Here's how the part is built. I have some questions about the finished solid (model axes, mm). Face numbers are marked on the shaded views. A direction names the side the tool comes from. Coordinates: 2 decimals unless noted, no trailing zeros. Write each loop counter-clockwise with the first axis right and the second up, starting at its lowest first coordinate (ties: lowest second). Pieces come first, ordered by that corner, then holes. Notation, with made-up numbers: (-4.5, -1) - (41.5, -1) arc R28 cw to (41.5, 32) - close; hole circle Ø8 at (-21.75, 9.25). An arc over 180 degrees is marked (long way). Answer in a Markdown table with one row per item. Add a question column.
Item 1: If I drill on probe 1 along X at (y, z) = (-10, -28); probe 2 along Z at (x, y) = (37, 12); probe 3 along Y at (x, z) = (90, -23), over which ranges is the centre line in solid material (lowest first)? Write a range as from..to.
Item 2: Imagine slicing it at A-A (y = 0). Please give me the cut outline in (x, z), plus the area to 3 significant figures.
Item 3: Imagine slicing it at C-C (x = 125.5). Please give me the cut outline in (y, z), plus the area to 3 significant figures.
Item 4: Imagine slicing it at D-D (y = 22). Please give me the cut outline in (x, z).
Item 5: Which directions (+Z, -Z, +X, -X, +Y, -Y) give clear straight access to the entire face, cutting with the end or side of a thin tool? Please do the marked faces 1 and 2.
Item 6: I'm going to push flat-ended pins straight in: pin 1 (12 mm diameter, centred on y = -4, z = -31, fed in from +X); pin 2 (6 mm diameter, centred on x = 84.5, z = 14, fed in from +Y); pin 3 (5 mm diameter, centred on x = 96.5, z = -17, fed in from -Y). Where does each tip first touch, or does it pass through?
from build123d import *

# Parameters (mm, degrees)
F0_R     = 40.5
F1_DEPTH = 100
F2_W     = 90
F2_H     = 90
F3_DEPTH = 100.001
F4_R     = 10
F5_DEPTH = 40


with BuildPart() as f1:
    # F0 (on Right) → F1 (new body)
    with BuildSketch(Plane.YZ):
        Circle(F0_R)
    extrude(amount=F1_DEPTH)

    # F2 (on face) → F3 (cut, through all)
    with BuildSketch(Plane.YZ.offset(100)):
        Rectangle(F2_W, F2_H)
        with BuildLine():
            Line((40, -6.3442887702), (40, -40))
            Line((40, -40), (6.3442887702, -40))
            ThreePointArc((6.3442887702, -40), (0, -40.5), (-6.3442887702, -40))
            Line((-6.3442887702, -40), (-40, -40))
            Line((-40, -40), (-40, -6.3442887702))
            ThreePointArc((-40, -6.3442887702), (-40.5, 0), (-40, 6.3442887702))
            Line((-40, 6.3442887702), (-40, 40))
            Line((-40, 40), (-6.3442887702, 40))
            ThreePointArc((-6.3442887702, 40), (0, 40.5), (6.3442887702, 40))
            Line((6.3442887702, 40), (40, 40))
            Line((40, 40), (40, 6.3442887702))
            ThreePointArc((40, 6.3442887702), (40.3748065011, 3.1819805153), (40.5, 0))
            ThreePointArc((40.5, 0), (40.3748065011, -3.1819805153), (40, -6.3442887702))
        make_face(mode=Mode.SUBTRACT)
        with BuildLine():
            ThreePointArc((-6.3442887702, -40), (0, -40.5), (6.3442887702, -40))
            Line((6.3442887702, -40), (-6.3442887702, -40))
        make_face()
        with BuildLine():
            Line((40, 6.3442887702), (40, -6.3442887702))
            ThreePointArc((40, -6.3442887702), (40.3748065011, -3.1819805153), (40.5, 0))
            ThreePointArc((40.5, 0), (40.3748065011, 3.1819805153), (40, 6.3442887702))
        make_face()
        with BuildLine():
            ThreePointArc((-40, 6.3442887702), (-40.5, 0), (-40, -6.3442887702))
            Line((-40, -6.3442887702), (-40, 6.3442887702))
        make_face()
        with BuildLine():
            Line((-6.3442887702, 40), (6.3442887702, 40))
            ThreePointArc((6.3442887702, 40), (0, 40.5), (-6.3442887702, 40))
        make_face()
    extrude(amount=-F3_DEPTH, mode=Mode.SUBTRACT)

    # F4 (on face) → F5 (join)
    with BuildSketch(Plane.YZ.offset(100)):
        Circle(F4_R)
    extrude(amount=F5_DEPTH)


solid = f1.part
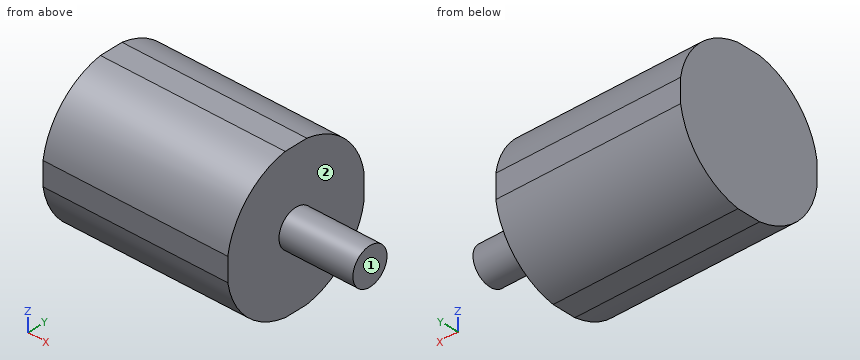
Here are the results:
| question | item | result |
|---|---|---|
| 1 | probe 1 | x = 0..100 |
| 1 | probe 2 | z = -38.68..38.68 |
| 1 | probe 3 | y = -33.34..33.34 |
| 2 | outline | (0, -40) - (100, -40) - (100, -10) - (140, -10) - (140, 10) - (100, 10) - (100, 40) - (0, 40) - close |
| 2 | area | 8,800 mm2 |
| 3 | outline | circle Ø20 at (0, 0) |
| 3 | area | 314 mm2 |
| 4 | outline | (0, -34) - (100, -34) - (100, 34) - (0, 34) - close |
| 5 | face 1 | +Z, -Z, +X, +Y, -Y |
| 5 | face 2 | +X |
| 6 | pin 1 | stops at x = 100 |
| 6 | pin 2 | stops at y = 38.98 |
| 6 | pin 3 | stops at y = -37.82 |
